Geometry check sheet. Reference: the model listing, model coordinates, mm. Face numbers are marked on the shaded views. A direction names the side the tool comes from. Round coordinates to 2 decimals unless told otherwise and drop trailing zeros. Loops run counter-clockwise (first coordinate to the right, second up) from the corner with the lowest first, then second, coordinate; pieces in that order, holes last. Notation, with made-up numbers: M 13,28 L 18,28 A30 ccw 18,53 Z; hole C -1.5,16 d1. An arc over 180 degrees is marked long. Use one line per item in the form item = value. Start each with the question number.
1. Cross-section at A-A (z = 0). Record the boundary of the cut face in (x, y).
2. Cross-section at D-D (y = 42.5). Record the boundary of the cut face in (x, z), then the cut area to 3 significant figures.
3. Go/stop test with flat-tipped pins: pin 1 (8 mm diameter, centred on x = 0.5, y = 17, fed in from -Z); pin 2 (1.3 mm diameter, centred on y = 54.5, z = -0.5, fed in from +X); pin 3 (1.5 mm diameter, centred on y = 28, z = 7.5, fed in from +X). Record where each tip stops, or that it passes through.
4. Material ranges on line 1 (Y direction, x = -1.75, z = 1.5); line 2 (Z direction, x = 0, y = 28); line 3 (Y direction, x = -8, z = -3), recorded low to high.
5. Cross-section at B-B (x = 0). Record the boundary of the cut face in (y, z).
6. Set-up check for the marked faces 1, 2 and 3: record each of +Z, -Z, +X, -X, +Y, -Y from which the full face is reachable in a straight line by a thin tool's end or side.
7. Cross-section at C-C (y = 3.5). Record the boundary of the cut face in (x, z), then the cut area to 3 significant figures.
```python
from build123d import *

# Parameters (mm, degrees)
SKETCH1_R                = 12.2
BOSS_EXTRUDE1_DEPTH      = 30.8
BOSS_EXTRUDE1_DEPTH_BACK = 1
FILLET2_R                = 1
SKETCH4_R                = 12.5
BOSS_EXTRUDE2_DEPTH      = 18
CHAMFER5_SIZE            = 2
CHAMFER5_SIZE2           = 0.069841539
SKETCH5_R                = 3.5
BOSS_EXTRUDE3_DEPTH      = 2.5
SKETCH6_R                = 2
BOSS_EXTRUDE4_DEPTH      = 1
BOSS_EXTRUDE6_DEPTH      = 8


with BuildPart() as part:
    # Sketch1 → Boss-Extrude1 (new body, two sides)
    with BuildSketch(Plane(origin=(0, 0, 0), x_dir=(1, 0, 0), z_dir=(0, 1, 0))) as boss_extrude1_sk:
        Circle(SKETCH1_R)
    extrude(amount=BOSS_EXTRUDE1_DEPTH)
    extrude(boss_extrude1_sk.sketch, amount=-BOSS_EXTRUDE1_DEPTH_BACK)

    # Fillet2
    fillet2_edges = [part.edges().sort_by_distance(p)[0] for p in [
        (-12.2, 30.8, 0),
    ]]
    fillet(fillet2_edges, radius=FILLET2_R)

    # Sketch4 → Boss-Extrude2 (add)
    with BuildSketch(Plane(origin=(0, 30.8, 0), x_dir=(1, 0, 0), z_dir=(0, 1, 0))):
        Circle(SKETCH4_R)
    extrude(amount=BOSS_EXTRUDE2_DEPTH)

    # Chamfer5
    chamfer5_edges = [part.edges().sort_by_distance(p)[0] for p in [
        (-12.5, 48.8, 0),
    ]]
    chamfer5_side = [part.faces().sort_by_distance(p)[0] for p in [
        (-12.5, 39.8, 0),
    ]]
    chamfer(chamfer5_edges, length=CHAMFER5_SIZE, length2=CHAMFER5_SIZE2, reference=chamfer5_side[0])

    # Sketch5 → Boss-Extrude3 (add)
    with BuildSketch(Plane(origin=(0, 48.8, 0), x_dir=(1, 0, 0), z_dir=(0, 1, 0))):
        Circle(SKETCH5_R)
    extrude(amount=BOSS_EXTRUDE3_DEPTH)

    # Sketch6 → Boss-Extrude4 (add)
    with BuildSketch(Plane(origin=(0, 51.3, 0), x_dir=(1, 0, 0), z_dir=(0, 1, 0))):
        Circle(SKETCH6_R)
    extrude(amount=BOSS_EXTRUDE4_DEPTH)

    # Sketch12 → Boss-Extrude6 (add)
    with BuildSketch(Plane(origin=(0, 52.3, 0), x_dir=(1, 0, 0), z_dir=(0, 1, 0))):
        with BuildLine():
            Line((1.5, 1.322875656), (1.5, -1.322875656))
            ThreePointArc((1.5, -1.322875656), (-2, 0), (1.5, 1.322875656))
        make_face()
    extrude(amount=BOSS_EXTRUDE6_DEPTH)


solid = part.part
```
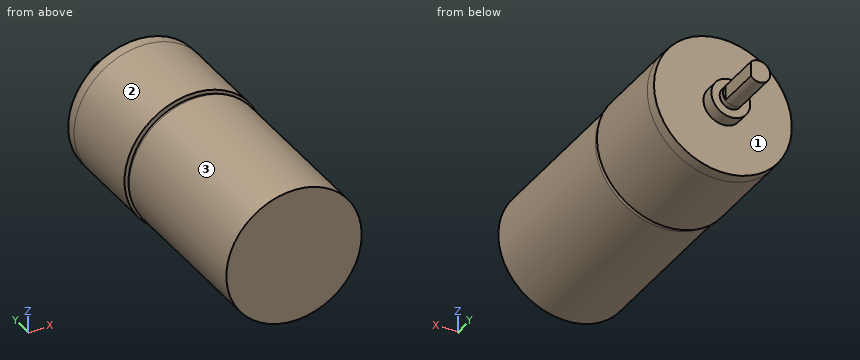
Reported:
q1.outline = M -12.5,30.8 L -11.2,30.8 A1 ccw -12.2,29.8 L -12.2,-1 L 12.2,-1 L 12.2,29.8 A1 ccw 11.2,30.8 L 12.5,30.8 L 12.5,46.8 L 12.43,48.8 L 3.5,48.8 L 3.5,51.3 L 2,51.3 L 2,52.3 L 1.5,52.3 L 1.5,60.3 L -2,60.3 L -2,51.3 L -3.5,51.3 L -3.5,48.8 L -12.43,48.8 L -12.5,46.8 Z
q2.outline = C 0,0 d25
q2.area = 491 mm²
q3.pin_1 = -12.2
q3.pin_2 = 1.5
q3.pin_3 = 10.16
q4.line_1 = -1 to 51.3
q4.line_2 = -12.2 to 12.2
q4.line_3 = -1 to 48.8
q5.outline = M -1,-12.2 L 29.8,-12.2 A1 ccw 30.8,-11.2 L 30.8,-12.5 L 46.8,-12.5 L 48.8,-12.43 L 48.8,-3.5 L 51.3,-3.5 L 51.3,-2 L 60.3,-2 L 60.3,2 L 51.3,2 L 51.3,3.5 L 48.8,3.5 L 48.8,12.43 L 46.8,12.5 L 30.8,12.5 L 30.8,11.2 A1 ccw 29.8,12.2 L -1,12.2 Z
q6.face_1 = +Y
q6.face_2 = +Y, -Y
q6.face_3 = -Y
q7.outline = C 0,0 d24.4
q7.area = 468 mm²
